Model file for the job. Use its own axes, mm. Coordinates: 2 decimals unless noted, no trailing zeros. Order: outer loops, then holes, each group sorted by start corner. A loop starts at its lowest first (then second) coordinate and runs counter-clockwise, first axis right, second up.
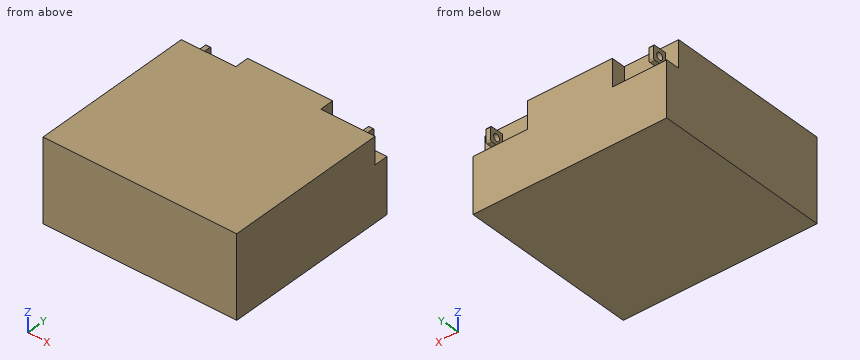
from build123d import *

# Parameters (mm, degrees)
SKETCH2_W           = 181.102
SKETCH2_H           = 76.962
BOSS_EXTRUDE1_DEPTH = 166.878
CUT_EXTRUDE1_DEPTH  = 194.722837699
SKETCH4_3_W         = 50.8
SKETCH4_3_H         = 25.4
CUT_EXTRUDE2_DEPTH  = 13.208
SKETCH5_W           = 4.318
SKETCH5_H           = 13.462
BOSS_EXTRUDE2_DEPTH = 13.208
SKETCH6_R           = 3.302
CUT_EXTRUDE3_DEPTH  = 13.208
FILLET1_R           = 1.27


with BuildPart() as part:
    # Sketch2 → Boss-Extrude1 (new body)
    with BuildSketch(Plane(origin=(0, 0, 0), x_dir=(1, 0, 0), z_dir=(0, 1, 0))):
        Rectangle(SKETCH2_W, SKETCH2_H)
    extrude(amount=BOSS_EXTRUDE1_DEPTH)

    # Sketch4 → Cut-Extrude1 (cut, through all)
    with BuildSketch(Plane(origin=(0, 166.878, 0), x_dir=(1, 0, 0), z_dir=(0, 1, 0))):
        Polygon((0, -38.481), (0, 0), (0, 38.481), (-90.551, 38.481), (-90.551, -38.481), align=None)
    extrude(amount=-CUT_EXTRUDE1_DEPTH, mode=Mode.SUBTRACT)

    # Sketch4<3> → Cut-Extrude2 (cut)
    with BuildSketch(Plane(origin=(0, 166.878, 0), x_dir=(1, 0, 0), z_dir=(0, 1, 0))):
        with Locations((65.151, -25.781)):
            Rectangle(SKETCH4_3_W, SKETCH4_3_H)
    extrude(amount=-CUT_EXTRUDE2_DEPTH, mode=Mode.SUBTRACT)

    # Sketch5 → Boss-Extrude2 (add)
    with BuildSketch(Plane(origin=(0, 153.67, 0), x_dir=(1, 0, 0), z_dir=(0, 1, 0))):
        with Locations((76.2, -25.781)):
            Rectangle(SKETCH5_W, SKETCH5_H)
    extrude(amount=BOSS_EXTRUDE2_DEPTH)

    # Sketch6 → Cut-Extrude3 (cut)
    with BuildSketch(Plane(origin=(78.359, 0, 0), x_dir=(0, 0, -1), z_dir=(1, 0, 0))):
        with Locations((-25.781, 160.274)):
            Circle(SKETCH6_R)
    extrude(amount=-CUT_EXTRUDE3_DEPTH, mode=Mode.SUBTRACT)

    # Fillet1
    fillet1_edges = [part.edges().sort_by_distance(p)[0] for p in [
        (76.2, 166.878, 32.512),
        (76.2, 166.878, 19.05),
    ]]
    fillet(fillet1_edges, radius=FILLET1_R)

    # Mirror1: part across plane


with BuildPart() as part_1:
    add(part.part)
    add(part.part.mirror(Plane.ZY))


solid = part_1.part
Q1. Probe line 1 (Y direction, x = -62, z = 14.5); line 2 (X direction, y = 158.5, z = 18). List the from-to ranges inside material, lowest first.
Established:
line 1: y = 0 to 153.67
line 2: x = -39.75 to 39.75
Q2. Cut at A-A, the plane x = -52.5. List the corners of the cut face in (y, z), plus the area to 3 significant figures.
Established:
outline: (0, -38.48) - (166.88, -38.48) - (166.88, 13.08) - (153.67, 13.08) - (153.67, 38.48) - (0, 38.48) - close
area: 12,500 mm2
Q3. Drop flat-ended pins along their axis: P1, Ø4, axis at y = 160.5, z = 23, coming from the +X side; P2, Ø2, axis at x = 77, y = 160.5, coming from the +Z side; P3, Ø4, axis at y = 158.5, z = 25, coming from the -X side. Give the stop position or say it passes through.
Established:
P1: stops at x = 78.36
P2: stops at z = 32.51
P3: stops at x = -78.36
